from build123d import *

# Parameters (mm, degrees)
F0_R          = 25.4
F1_DEPTH      = 43.18
F2_R          = 3.81
F3_DEPTH      = 43.181
F4_R          = 3.81
F5_DEPTH      = 25.401
F5_DEPTH_BACK = 25.401
F6_R          = 3.81
F7_DEPTH      = 25.4010001
F7_DEPTH_BACK = 25.4010001
F8_R          = 3.302
F9_DEPTH      = 43.1810001
F10_R         = 22.352
F11_DEPTH     = 40.64


with BuildPart() as f1:
    # F0 (on Top) → F1 (new body)
    with BuildSketch(Plane.XY):
        Circle(F0_R)
    extrude(amount=-F1_DEPTH)

    # F2 (on face) → F3 (cut, through all)
    with BuildSketch(Plane(origin=(0, 0, -43.18), x_dir=(1, 0, 0), z_dir=(0, 0, -1))):
        Circle(F2_R)
    extrude(amount=-F3_DEPTH, mode=Mode.SUBTRACT)

    # F4 (on Right) → F5 (cut, two sides)
    with BuildSketch(Plane.YZ) as f5_sk:
        with Locations((0, -10.16)):
            Circle(F4_R)
    extrude(amount=-F5_DEPTH, mode=Mode.SUBTRACT)
    extrude(f5_sk.sketch, amount=F5_DEPTH_BACK, mode=Mode.SUBTRACT)

    # F6 (on Front) → F7 (cut, two sides)
    with BuildSketch(Plane.XZ) as f7_sk:
        with Locations((0, -10.16)):
            Circle(F6_R)
    extrude(amount=-F7_DEPTH, mode=Mode.SUBTRACT)
    extrude(f7_sk.sketch, amount=F7_DEPTH_BACK, mode=Mode.SUBTRACT)

    # F8 (on face) → F9 (cut, through all)
    with BuildSketch(Plane(origin=(0, 0, -43.18), x_dir=(1, 0, 0), z_dir=(0, 0, -1))):
        with Locations((10.9096324106, 0)):
            Circle(F8_R)
        with Locations((-10.8710342307, 0)):
            Circle(F8_R)
    extrude(amount=-F9_DEPTH, mode=Mode.SUBTRACT)

    # F10 (on face) → F11 (cut)
    with BuildSketch(Plane.XY):
        Circle(F10_R)
    extrude(amount=-F11_DEPTH, mode=Mode.SUBTRACT)


solid = f1.part
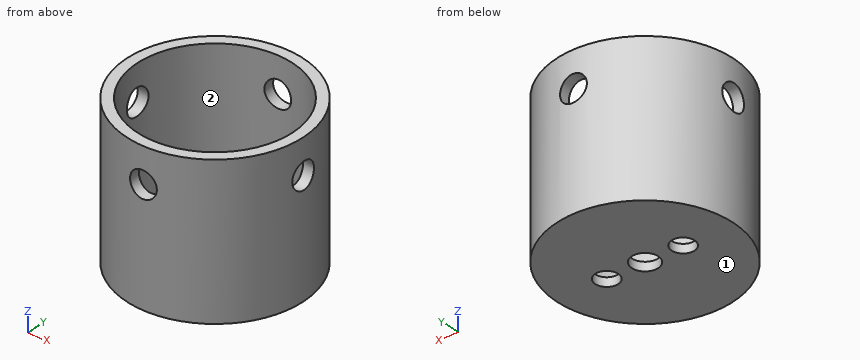
Input: part model. Units: mm. Frame: model coordinates. Face numbers are marked on the shaded views. A direction names the side the tool comes from. Round coordinates to 2 decimals unless told otherwise and drop trailing zeros. Write each loop counter-clockwise with the first axis right and the second up, starting at its lowest first coordinate (ties: lowest second). Pieces come first, ordered by that corner, then holes.
1) Cut plane B-B (x = 0). Return the cut outline in (y, z).
2) Contact query for flat-ended pins moving along their axis: P1, Ø10, axis at y = 0, z = -10.16, coming from the +X side; P2, Ø9, axis at x = 0, y = 0, coming from the +Z side; P3, Ø4, axis at x = -19.5, z = -18.5, coming from the +Y side; P4, Ø1, axis at y = -18, z = -20.5, coming from the -X side. Output: stop coordinate, or through.
3) Cut plane D-D (x = -9). Return the cut outline in (y, z).
4) Cut plane A-A (y = 0). Return the cut outline in (x, z).
5) Reachability of the marked faces 1 and 2 from +Z, -Z, +X, -X, +Y, -Y: full face, straight path, thin tool, end or side. Return the list, or none.
6) Ray query, L1, parallel to X at y = 0, z = -41.25; L2, parallel to Y at x = -0.5, z = -36; L3, parallel to Z at x = 23.2, y = 0. Return the intervals inside material, ascending.
7) Cut plane C-C (z = -7.5). Return the cut outline in (x, y).
Geometry says:
1. outline: (-25.4, -43.18) - (-3.81, -43.18) - (-3.81, -40.64) - (-22.35, -40.64) - (-22.35, -13.97) - (-25.4, -13.97) - close; (-25.4, -6.35) - (-22.35, -6.35) - (-22.35, 0) - (-25.4, 0) - close; (3.81, -43.18) - (25.4, -43.18) - (25.4, -13.97) - (22.35, -13.97) - (22.35, -40.64) - (3.81, -40.64) - close; (22.35, -6.35) - (25.4, -6.35) - (25.4, 0) - (22.35, 0) - close
2. P1: stops at x = 25.4
2. P2: stops at z = -40.64
2. P3: stops at y = 18.41
2. P4: stops at x = -18.41
3. outline: (-23.75, -43.18) - (-2.72, -43.18) - (-2.72, -40.64) - (-20.46, -40.64) - (-20.46, 0) - (-23.75, 0) - close; (2.72, -43.18) - (23.75, -43.18) - (23.75, 0) - (20.46, 0) - (20.46, -40.64) - (2.72, -40.64) - close
4. outline: (-25.4, -43.18) - (-14.17, -43.18) - (-14.17, -40.64) - (-22.35, -40.64) - (-22.35, -13.97) - (-25.4, -13.97) - close; (-25.4, -6.35) - (-22.35, -6.35) - (-22.35, 0) - (-25.4, 0) - close; (-7.57, -43.18) - (-3.81, -43.18) - (-3.81, -40.64) - (-7.57, -40.64) - close; (3.81, -43.18) - (7.61, -43.18) - (7.61, -40.64) - (3.81, -40.64) - close; (14.21, -43.18) - (25.4, -43.18) - (25.4, -13.97) - (22.35, -13.97) - (22.35, -40.64) - (14.21, -40.64) - close; (22.35, -6.35) - (25.4, -6.35) - (25.4, 0) - (22.35, 0) - close
5. face 1: -Z, +X, -X, +Y, -Y
5. face 2: +Z
6. L1: x = -25.4 to -14.17, -7.57 to -3.81, 3.81 to 7.61, 14.21 to 25.4
6. L2: y = -25.4 to -22.35, 22.35 to 25.4
6. L3: z = -43.18 to -13.97, -6.35 to 0
7. outline: (-25.25, -2.73) arc R25.4 ccw to (-2.73, -25.25) - (-2.73, -22.18) arc R22.35 cw to (-22.18, -2.73) - close; (-25.25, 2.73) - (-22.18, 2.73) arc R22.35 cw to (-2.73, 22.18) - (-2.73, 25.25) arc R25.4 ccw to start; (2.73, -25.25) arc R25.4 ccw to (25.25, -2.73) - (22.18, -2.73) arc R22.35 cw to (2.73, -22.18) - close; (2.73, 22.18) arc R22.35 cw to (22.18, 2.73) - (25.25, 2.73) arc R25.4 ccw to (2.73, 25.25) - close
